```python
from build123d import *

# Parameters (mm, degrees)
SKETCH1_W           = 20
SKETCH1_H           = 50
BOSS_EXTRUDE1_DEPTH = 12.525
SKETCH2_W           = 20
SKETCH2_H           = 3.75
BOSS_EXTRUDE2_DEPTH = 10
CUT_EXTRUDE1_DEPTH  = 2.75
SKETCH5_R           = 0.8
CUT_EXTRUDE2_DEPTH  = 28.25
FILLET1_R           = 0.4
FILLET2_R           = 3
SKETCH6_W           = 20
SKETCH6_H           = 20
CUT_EXTRUDE3_DEPTH  = 10.025
SKETCH7_R           = 3.01
CUT_EXTRUDE4_DEPTH  = 3.5
BOSS_EXTRUDE3_DEPTH = 2.5
CUT_EXTRUDE6_DEPTH  = 10.025
SKETCH13_W          = 20
SKETCH13_H          = 6.249999854
CUT_EXTRUDE8_DEPTH  = 23.525
SKETCH14_W          = 30
SKETCH14_H          = 10
BOSS_EXTRUDE4_DEPTH = 2.5
CUT_EXTRUDE7_DEPTH  = 3.5
FILLET3_R           = 2
FILLET4_R           = 2.5
SKETCH15_R          = 9
CUT_EXTRUDE10_DEPTH = 21.025


with BuildPart() as part:
    # Sketch1 → Boss-Extrude1 (new body)
    with BuildSketch(Plane(origin=(0, 0, 0), x_dir=(1, 0, 0), z_dir=(0, 1, 0))):
        Rectangle(SKETCH1_W, SKETCH1_H)
    extrude(amount=BOSS_EXTRUDE1_DEPTH)

    # Sketch2 → Boss-Extrude2 (add)
    with BuildSketch(Plane(origin=(0, 12.525, 0), x_dir=(1, 0, 0), z_dir=(0, 1, 0))):
        with Locations((0, -3.125)):
            Rectangle(SKETCH2_W, SKETCH2_H)
    extrude(amount=BOSS_EXTRUDE2_DEPTH)

    # Sketch3 → Cut-Extrude1 (cut)
    with BuildSketch(Plane.XY.offset(5)):
        with BuildLine():
            Line((-4, 19.025), (-4, 22.525))
            Line((-4, 22.525), (4, 22.525))
            Line((4, 22.525), (4, 19.025))
            Line((4, 19.025), (4.5, 19.025))
            ThreePointArc((4.5, 19.025), (6, 17.525), (4.5, 16.025))
            Line((4.5, 16.025), (3.708099244, 16.025))
            ThreePointArc((3.708099244, 16.025), (0, 13.525), (-3.708099244, 16.025))
            Line((-3.708099244, 16.025), (-4.5, 16.025))
            ThreePointArc((-4.5, 16.025), (-6, 17.525), (-4.5, 19.025))
            Line((-4.5, 19.025), (-4, 19.025))
        make_face()
    extrude(amount=-CUT_EXTRUDE1_DEPTH, mode=Mode.SUBTRACT)

    # Sketch5 → Cut-Extrude2 (cut, through all)
    with BuildSketch(Plane.XY.offset(2.25)):
        with Locations((-4.5, 17.525)):
            Circle(SKETCH5_R)
        with Locations((4.5, 17.525)):
            Circle(SKETCH5_R)
        with BuildLine():
            Line((-2.25, 17.525), (-2.25, 22.525))
            Line((-2.25, 22.525), (2.25, 22.525))
            Line((2.25, 22.525), (2.25, 17.525))
            ThreePointArc((2.25, 17.525), (0, 15.275), (-2.25, 17.525))
        make_face()
    extrude(amount=-CUT_EXTRUDE2_DEPTH, mode=Mode.SUBTRACT)

    # Fillet1
    fillet1_edges = [part.edges().sort_by_distance(p)[0] for p in [
        (3.708099244, 16.025, 3.625),
        (-3.708099244, 16.025, 3.625),
        (-4, 19.025, 3.625),
        (4, 19.025, 3.625),
        (0, 13.525, 2.25),
        (-4.104049622, 16.025, 2.25),
        (-6, 17.525, 2.25),
        (-4.25, 19.025, 2.25),
        (-4, 20.775, 2.25),
        (4, 20.775, 2.25),
        (4.25, 19.025, 2.25),
        (6, 17.525, 2.25),
        (4.104049622, 16.025, 2.25),
    ]]
    fillet(fillet1_edges, radius=FILLET1_R)

    # Fillet2
    fillet2_edges = [part.edges().sort_by_distance(p)[0] for p in [
        (10, 22.525, 3.125),
        (-10, 22.525, 3.125),
    ]]
    fillet(fillet2_edges, radius=FILLET2_R)

    # Sketch6 → Cut-Extrude3 (cut)
    with BuildSketch(Plane(origin=(0, 12.525, 0), x_dir=(1, 0, 0), z_dir=(0, 1, 0))):
        with Locations((0, -15)):
            Rectangle(SKETCH6_W, SKETCH6_H)
    extrude(amount=-CUT_EXTRUDE3_DEPTH, mode=Mode.SUBTRACT)

    # Sketch7 → Cut-Extrude4 (cut, through all)
    with BuildSketch(Plane(origin=(0, 2.5, 0), x_dir=(1, 0, 0), z_dir=(0, 1, 0))):
        with Locations((0, -13.750000146)):
            Circle(SKETCH7_R)
    extrude(amount=-CUT_EXTRUDE4_DEPTH, mode=Mode.SUBTRACT)

    # Sketch8 → Boss-Extrude3 (add)
    with BuildSketch(Plane.ZY.offset(10)):
        with BuildLine():
            Line((5, 2.5), (22.025, 2.5))
            ThreePointArc((22.025, 2.5), (9.98650705, 7.48650705), (5, 19.525))
            Line((5, 19.525), (5, 2.5))
        make_face()
        with BuildLine():
            Line((1.25, 12.525), (-5.75, 12.525))
            ThreePointArc((-5.75, 12.525), (-0.800252532, 14.575252532), (1.25, 19.525))
            Line((1.25, 19.525), (1.25, 12.525))
        make_face()
    boss_extrude3 = extrude(amount=-BOSS_EXTRUDE3_DEPTH)

    # Sketch11 → Cut-Extrude6 (cut)
    with BuildSketch(Plane(origin=(0, 12.525, 0), x_dir=(1, 0, 0), z_dir=(0, 1, 0))):
        with BuildLine():
            Line((-3.65, 25), (-10, 25))
            Line((-10, 25), (-10, 8))
            ThreePointArc((-10, 8), (-5.509871939, 9.859871939), (-3.65, 14.35))
            Line((-3.65, 14.35), (-3.65, 25))
        make_face()
    cut_extrude6 = extrude(amount=-CUT_EXTRUDE6_DEPTH, mode=Mode.SUBTRACT)

    # Mirror1: Boss-Extrude3, Cut-Extrude6 across plane
    add(boss_extrude3.mirror(Plane(origin=(0, 0, 0), x_dir=(0, 0, 1), z_dir=(1, 0, 0))))
    add(cut_extrude6.mirror(Plane(origin=(0, 0, 0), x_dir=(0, 0, 1), z_dir=(1, 0, 0))), mode=Mode.SUBTRACT)

    # Sketch13 → Cut-Extrude8 (cut, through all)
    with BuildSketch(Plane.XZ):
        with Locations((0, 21.875000073)):
            Rectangle(SKETCH13_W, SKETCH13_H)
    extrude(amount=-CUT_EXTRUDE8_DEPTH, mode=Mode.SUBTRACT)

    # Sketch14 → Boss-Extrude4 (add)
    with BuildSketch(Plane.XZ):
        with Locations((0, 5.740000146)):
            Rectangle(SKETCH14_W, SKETCH14_H)
    extrude(amount=-BOSS_EXTRUDE4_DEPTH)

    # Sketch12 → Cut-Extrude7 (cut, through all)
    with BuildSketch(Plane(origin=(0, 2.5, 0), x_dir=(1, 0, 0), z_dir=(0, 1, 0))):
        with BuildLine():
            Line((-5, 21.5), (-5, 18.5))
            ThreePointArc((-5, 18.5), (-6.5, 17), (-8, 18.5))
            Line((-8, 18.5), (-8, 21.5))
            ThreePointArc((-8, 21.5), (-6.5, 23), (-5, 21.5))
        make_face()
        with BuildLine():
            Line((8, 21.5), (8, 18.5))
            ThreePointArc((8, 18.5), (6.5, 17), (5, 18.5))
            Line((5, 18.5), (5, 21.5))
            ThreePointArc((5, 21.5), (6.5, 23), (8, 21.5))
        make_face()
        with BuildLine():
            Line((-14, -7.240000146), (-14, -4.240000146))
            ThreePointArc((-14, -4.240000146), (-12.5, -2.740000146), (-11, -4.240000146))
            Line((-11, -4.240000146), (-11, -7.240000146))
            ThreePointArc((-11, -7.240000146), (-12.5, -8.740000146), (-14, -7.240000146))
        make_face()
        with BuildLine():
            Line((11, -7.240000146), (11, -4.240000146))
            ThreePointArc((11, -4.240000146), (12.5, -2.740000146), (14, -4.240000146))
            Line((14, -4.240000146), (14, -7.240000146))
            ThreePointArc((14, -7.240000146), (12.5, -8.740000146), (11, -7.240000146))
        make_face()
    extrude(amount=-CUT_EXTRUDE7_DEPTH, mode=Mode.SUBTRACT)

    # Fillet3
    fillet3_edges = [part.edges().sort_by_distance(p)[0] for p in [
        (-10, 1.25, -25),
        (10, 1.25, -25),
        (15, 1.25, 0.740000146),
        (-15, 1.25, 10.740000146),
        (-10, 1.25, 10.740000146),
        (10, 1.25, 10.740000146),
        (-15, 1.25, 0.740000146),
        (10, 1.25, 0.740000146),
        (-10, 1.25, 0.740000146),
        (15, 1.25, 10.740000146),
    ]]
    fillet(fillet3_edges, radius=FILLET3_R)

    # Fillet4
    fillet4_edges = [part.edges().sort_by_distance(p)[0] for p in [
        (10, 1.408982762, 18.750000146),
        (-10, 1.408982762, 18.750000146),
    ]]
    fillet(fillet4_edges, radius=FILLET4_R)

    # Sketch15 → Cut-Extrude10 (cut, through all)
    with BuildSketch(Plane(origin=(0, 2.5, 0), x_dir=(1, 0, 0), z_dir=(0, 1, 0))):
        with Locations((0, -13.750000146)):
            Circle(SKETCH15_R)
    extrude(amount=CUT_EXTRUDE10_DEPTH, mode=Mode.SUBTRACT)


solid = part.part
```
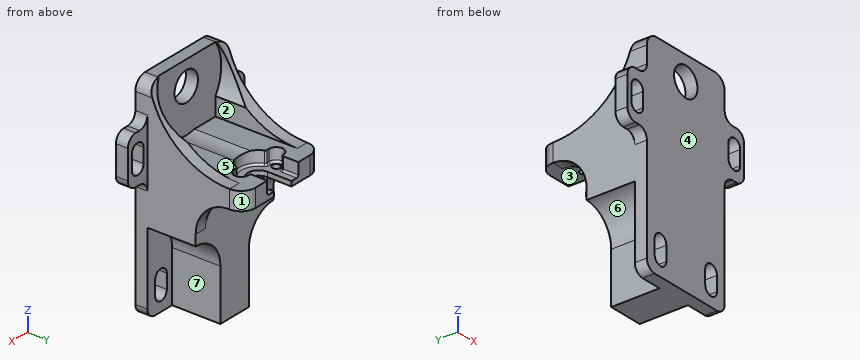
Input: part model. Units: mm. Frame: model coordinates. Face numbers are marked on the shaded views. A direction names the side the tool comes from. Coordinates: 2 decimals unless noted, no trailing zeros. Write each loop counter-clockwise with the first axis right and the second up, starting at its lowest first coordinate (ties: lowest second). Pieces come first, ordered by that corner, then holes. Notation, with made-up numbers: (-14, 55.25) - (11, 55.25) arc R26 ccw to (11, 77.25) - close; hole circle Ø7 at (24.5, 41.25). An arc over 180 degrees is marked (long way). Put each result on its own line as item: value. Start each with the question number.
1) Contact query for flat-ended pins moving along their axis: pin 1 (2 mm diameter, centred on x = -2.5, y = 7.5, fed in from +Z); pin 2 (8 mm diameter, centred on y = 11, z = 8.5, fed in from -X); pin 3 (5 mm diameter, centred on y = 7.5, z = -22, fed in from +X); pin 4 (12 mm diameter, centred on x = 4.5, z = -4, fed in from -Y). Output: stop coordinate, or through.
2) Cut plane C-C (z = 15.5). Return the cut outline in (x, y).
3) Cut plane A-A (y = 11.5). Return the cut outline in (x, z), plus the area to 3 significant figures.
4) Ray query, L1, parallel to X at y = 5, z = 7; L2, parallel to Y at x = -4.5, z = 1.75 (3 decimals); L3, parallel to Z at x = 0, y = 0.7. Return the intervals inside material, ascending.
5) Reachability of the marked faces 5, 6 and 7 from +Z, -Z, +X, -X, +Y, -Y: full face, straight path, thin tool, end or side. Return the list, or none.
6) Cut plane B-B (x = 6.5). Return the cut outline in (y, z) (3 decimals), plus the area to 3 significant figures.
7) Cut plane D-D (z = -22). Return the cut outline in (x, y) (3 decimals).
8) Mould query, pull axis X, two halves, no side actions, for the marked faces 1, 2, 3 and 4. Classes: pulls with the +X half, pulls with the -X half, needs draft (parallel to the pull), parting line crosses it, or undercut.
Resolved:
1. pin 1: stops at z = 5
1. pin 2: stops at x = -10
1. pin 3: stops at x = 3.65
1. pin 4: stops at y = 0
2. outline: (-10, 0) - (-2.45, 0) - (-2.45, 2.5) - (-8.83, 2.5) - (-8.83, 3.8) - (-10, 3.8) - close; (2.45, 0) - (10, 0) - (10, 3.8) - (8.83, 3.8) - (8.83, 2.5) - (2.45, 2.5) - close
3. outline: (-10, -8) arc R6.35 cw to (-3.65, -14.35) - (-3.65, -25) - (3.65, -25) - (3.65, -14.35) arc R6.35 cw to (10, -8) - (10, 7.01) - (7.5, 7.01) - (7.5, 5) - (2.11, 5) arc R9 cw to (-2.11, 5) - (-7.5, 5) - (-7.5, 7.01) - (-10, 7.01) - close
3. area: 411 mm2
4. L1: x = -10 to -7.5, 7.5 to 10
4. L2: y = 0 to 16.725, 18.325 to 22.525
4. L3: z = -25 to 10.74, 16.76 to 18.75
5. face 5: +Z, +Y
5. face 6: -Z, -X, +Y
5. face 7: -Z, +X, +Y
6. outline: (0, -25) - (2.5, -25) - (2.5, -23) - (0, -23) - close; (0, -17) - (2.5, -17) - (2.5, -9.052) - (12.525, -9.052) - (12.525, 1.25) - (22.525, 1.25) - (22.525, 5) - (2.5, 5) - (2.5, 18.75) - (0, 18.75) - close
6. area: 273 mm2
7. outline: (-10, 0) - (-7.914, 0) - (-7.914, 2.5) - (-10, 2.5) - close; (-5.086, 0) - (5.086, 0) - (5.086, 2.5) - (3.65, 2.5) - (3.65, 12.525) - (-3.65, 12.525) - (-3.65, 2.5) - (-5.086, 2.5) - close; (7.914, 0) - (10, 0) - (10, 2.5) - (7.914, 2.5) - close
8. face 1: pulls with the +X half
8. face 2: undercut
8. face 3: undercut
8. face 4: needs draft
